CAD build for the part. Positions are in the model's coordinates, mm. A direction names the side the tool comes from. Coordinates: 2 decimals unless noted, no trailing zeros. Order: outer loops, then holes, each group sorted by start corner. A loop starts at its lowest first (then second) coordinate and runs counter-clockwise, first axis right, second up. Notation, with made-up numbers: (-37.75, 5.25) - (14.25, 5.25) arc R20 cw to (14.25, 29.25) - close; hole circle Ø8 at (-5.5, -1.75). An arc over 180 degrees is marked (long way). Use one line per item in the form item = value.
```python
from build123d import *

# Parameters (mm, degrees)
SKETCH1_R                = 35.5
SKETCH1_R_2              = 32.5
BOSS_EXTRUDE1_DEPTH      = 63
SKETCH2_R                = 32.5
BOSS_EXTRUDE2_DEPTH      = 3
BOSS_EXTRUDE6_DEPTH      = 14.275
BOSS_EXTRUDE6_DEPTH_BACK = 11.725
SKETCH7_R                = 13
BOSS_EXTRUDE7_DEPTH      = 6
SKETCH8_R                = 10
CUT_EXTRUDE1_DEPTH       = 3
SKETCH9_R                = 1.275
CUT_EXTRUDE2_DEPTH       = 67.65770114


with BuildPart() as part:
    # Sketch1 → Boss-Extrude1 (new body)
    with BuildSketch(Plane.XY):
        Circle(SKETCH1_R)
        Circle(SKETCH1_R_2, mode=Mode.SUBTRACT)
    extrude(amount=BOSS_EXTRUDE1_DEPTH)

    # Sketch2 → Boss-Extrude2 (add)
    with BuildSketch(Plane(origin=(0, 0, 0), x_dir=(-1, 0, 0), z_dir=(0, 0, -1))):
        Circle(SKETCH2_R)
    extrude(amount=-BOSS_EXTRUDE2_DEPTH)

    # Sketch6 → Boss-Extrude6 (add, two sides)
    with BuildSketch(Plane.XY.offset(26.896958138)) as boss_extrude6_sk:
        with BuildLine():
            Line((-34.208935101, 9.486767586), (-102.85732032, -27.128564879))
            Line((-102.85732032, -27.128564879), (-100.033619175, -32.422590931))
            Line((-100.033619175, -32.422590931), (-35.441970042, 2.028979924))
            ThreePointArc((-35.441970042, 2.028979924), (-35.024517071, 5.790786127), (-34.208935101, 9.486767586))
        make_face()
    extrude(amount=BOSS_EXTRUDE6_DEPTH)
    extrude(boss_extrude6_sk.sketch, amount=-BOSS_EXTRUDE6_DEPTH_BACK)

    # Sketch7 → Boss-Extrude7 (add)
    with BuildSketch(Plane(origin=(-8.692215236, 16.296630393, 0), x_dir=(0.882337675, 0.470616858, 0), z_dir=(0.470616858, -0.882337675, 0))):
        with Locations((-103.522048859, 28.171958138)):
            Circle(SKETCH7_R)
    extrude(amount=-BOSS_EXTRUDE7_DEPTH)

    # Sketch8 → Cut-Extrude1 (cut)
    with BuildSketch(Plane(origin=(-11.515916381, 21.590656445, 0), x_dir=(0.882337675, 0.470616858, 0), z_dir=(-0.470616858, 0.882337675, 0))):
        with Locations((-103.522048859, -28.171958138)):
            Circle(SKETCH8_R)
    extrude(amount=-CUT_EXTRUDE1_DEPTH, mode=Mode.SUBTRACT)

    # Sketch9 → Cut-Extrude2 (cut, through all)
    with BuildSketch(Plane(origin=(-8.692215236, 16.296630393, 0), x_dir=(0.882337675, 0.470616858, 0), z_dir=(0.470616858, -0.882337675, 0))):
        with Locations((-103.522048859, 35.171958138)):
            Circle(SKETCH9_R)
        with Locations((-110.522048859, 28.171958138)):
            Circle(SKETCH9_R)
        with Locations((-96.522048859, 28.171958138)):
            Circle(SKETCH9_R)
        with Locations((-103.522048859, 21.171958138)):
            Circle(SKETCH9_R)
    extrude(amount=-CUT_EXTRUDE2_DEPTH, mode=Mode.SUBTRACT)


solid = part.part
```
Item 1: Cut at C-C, the plane z = 13.5. Write the cut outline in (x, y), plus the area to 3 significant figures.
Derived:
outline = circle Ø71 at (0, 0); hole circle Ø65 at (0, 0)
area = 641 mm²
Item 2: Drop flat-ended pins along their axis: pin 1 (12 mm diameter, centred on x = -92.5, z = 33, fed in from +Y); pin 2 (12 mm diameter, centred on x = -17.5, z = 25.5, fed in from -Y); pin 3 (8 mm diameter, centred on x = -76.5, y = -21.5, fed in from -Z). Give the stop position or say it passes through.
Derived:
pin_1 = -18.4
pin_2 = -33.59
pin_3 = 15.17
Item 3: Two-plate mould, pull along Y, no slides. Class faces 1 (the face through (31, 9.76, 32.58)), 2 (the face through (-112.893, -35.929, 28.458)), 3 (the face through (0, 0, 0)): +Y half, -Y half, draft (parallel to the pull), parting line (faces both ways), or undercut.
Derived:
face_1 = undercut
face_2 = -Y half
face_3 = draft
Item 4: Cut at B-B, the plane x = 0. Write the cut outline in (y, z).
Derived:
outline = (-35.5, 0) - (35.5, 0) - (35.5, 63) - (32.5, 63) - (32.5, 3) - (-32.5, 3) - (-32.5, 63) - (-35.5, 63) - close
Item 5: Drill centre lines: line 1 (Y direction, x = 0, z = 49.5); line 2 (X direction, y = -29.5, z = 38.5); line 3 (X direction, y = -27, z = 41). Where is each one in solid material? Low to high. Write a range as [from, to].
Derived:
line_1 = [-35.5, -32.5], [32.5, 35.5]
line_2 = [-107.3, -94.55], [-19.75, -13.64], [13.64, 19.75]
line_3 = [-102.62, -89.87], [-23.05, -18.09], [18.09, 23.05]
Item 6: Cut at A-A, the plane y = 0. Write the cut outline in (x, z), plus the area to 3 significant figures.
Derived:
outline = (-52, 15.17) - (-39.25, 15.17) - (-39.25, 41.17) - (-52, 41.17) - close; (-35.5, 0) - (35.5, 0) - (35.5, 63) - (32.5, 63) - (32.5, 3) - (-32.5, 3) - (-32.5, 63) - (-35.5, 63) - close
area = 904 mm²
Item 7: Cut at D-D, the plane y = 20. Write the cut outline in (x, z), plus the area to 3 significant figures.
Derived:
outline = (-29.33, 0) - (29.33, 0) - (29.33, 63) - (25.62, 63) - (25.62, 3) - (-25.62, 3) - (-25.62, 63) - (-29.33, 63) - close
area = 621 mm²
Item 8: 3-axis set-ups, long thin cutter, end or side, ignore diameter. For faces 4 (the face through (0, 0, 3)), 5 (the face through (16, -29, 63)), 6 (the face through (-101.57, -29.84, 28.03)): which of +Z, -Z, +X, -X, +Y, -Y reach the whole face in a straight line?
Derived:
face_4 = +Z
face_5 = +Z, +X, -X, +Y, -Y
face_6 = none
